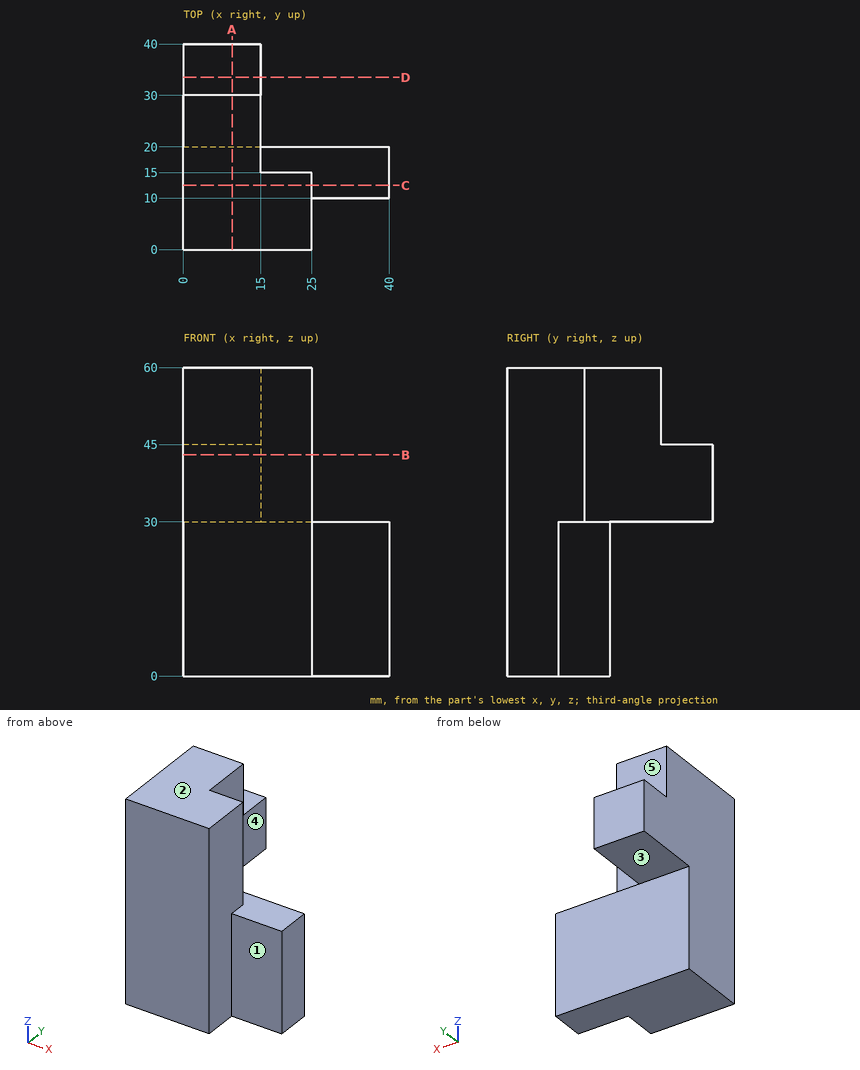
Check sheet for the drawn part. Datum: minimum x, y, z corner. Units: mm. A direction names the side the tool comes from. Round coordinates to 2 decimals unless told otherwise and drop trailing zeros. Order: outer loops, then holes, each group sorted by start corner. A loop starts at its lowest first (then second) coordinate and runs counter-clockwise, first axis right, second up.
1) Section check B-B (z = 43). Record the boundary of the cut face in (x, y), and give its area (3 significant figures).
2) Tool access check on the marked faces 1, 2, 3, 4 and 5. Record the directions out of +Z, -Z, +X, -X, +Y, -Y that give a thin tool (end or side, any length) a straight path to the whole face; none if there is none.
3) Go/stop test with flat-tipped pins: pin 1 Ø7.5 at (x, z) = (32, 12.5) entering from -Y; pin 2 Ø7.5 at (x, y) = (6, 28) entering from -Z; pin 3 Ø6 at (x, y) = (19.5, 27.5) entering from -Z; pin 4 Ø5 at (x, z) = (20.5, 43) entering from +Y. Record where each tip stops, or that it passes through.
4) Section check C-C (y = 12.5). Record the boundary of the cut face in (x, z).
5) Scan lines: line 1 (Y direction, x = 6, z = 29); line 2 (X direction, y = 8, z = 35); line 3 (Y direction, x = 37, z = 8). Record each from-to range of solid material in increasing order.
6) Section check A-A (x = 9.5). Record the boundary of the cut face in (y, z).
7) Section check D-D (y = 33.5). Record the boundary of the cut face in (x, z).
Result:
1. outline: (0, 0) - (25, 0) - (25, 15) - (15, 15) - (15, 40) - (0, 40) - close
1. area: 750 mm2
2. face 1: +Z, -Z, +X, -Y
2. face 2: +Z, +X, -X, +Y, -Y
2. face 3: -Z, +X, -X, +Y
2. face 4: +Z, +X, +Y
2. face 5: +Z, +X, -X, +Y
3. pin 1: stops at y = 10
3. pin 2: stops at z = 30
3. pin 3: passes through
3. pin 4: stops at y = 15
4. outline: (0, 0) - (40, 0) - (40, 30) - (25, 30) - (25, 60) - (0, 60) - close
5. line 1: y = 0 to 20
5. line 2: x = 0 to 25
5. line 3: y = 10 to 20
6. outline: (0, 0) - (20, 0) - (20, 30) - (40, 30) - (40, 45) - (30, 45) - (30, 60) - (0, 60) - close
7. outline: (0, 30) - (15, 30) - (15, 45) - (0, 45) - close
